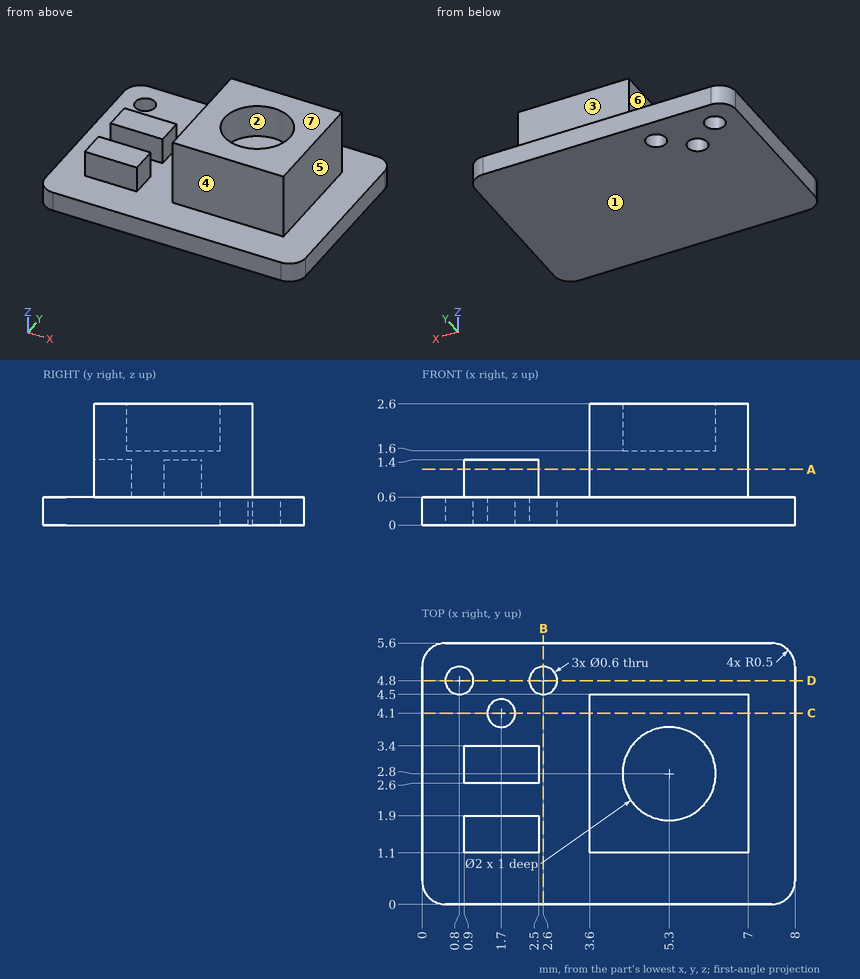
Answer from the drawing. Dimensions are ordinates in mm from the lowest x, y and z of the part. A direction names the side the tool comes from. Give positions to 0.01 mm unless a question says otherwise; leave off trailing zeros. Write each loop counter-clockwise with the first axis right and the second up, starting at its lowest first coordinate (ties: lowest second). Pieces come first, ordered by that corner, then holes.
1) Section A-A (z = 1.2) is taken. Write down the section's boundary in (x, y), and give its area (3 significant figures).
2) Section D-D (y = 4.8) is taken. Write down the section's boundary in (x, z), and give its area (3 significant figures).
3) A tool of negligible diameter and unlimited length cuts with its end or side. For the marked faces 4, 5, 6 and 7, from which of +Z, -Z, +X, -X, +Y, -Y can it reach the whole face along a straight path? Write none if from no direction.
4) Section C-C (y = 4.1) is taken. Write down the section's boundary in (x, z).
5) Section B-B (x = 2.6) is taken. Write down the section's boundary in (y, z).
6) Find the intervals of material crossed by L1, parallel to X at y = 4.8, z = 0.35; L2, parallel to X at y = 4.1, z = 0.45; L3, parallel to Y at x = 5.3, z = 1.9, in increasing order.
7) For a pull along Y with two mould halves and no side action, classify the marked faces 1, 2 and 3 as pulls with the +Y half, pulls with the -Y half, needs draft (parallel to the pull), parting line crosses it, or undercut.
8) Given P1, Ø0.9, axis at x = 2, y = 3, coming from the +Z side; P2, Ø0.6, axis at y = 3, z = 1, coming from the -X side; P3, Ø1, axis at y = 3.5, z = 1, coming from the -X side; P4, Ø0.6, axis at x = 1.5, z = 1, coming from the +Y side, each flat-ended and moving along its own axis, determine where each tip first touches the part or whether it passes through.
Response:
1. outline: (0.9, 1.1) - (2.5, 1.1) - (2.5, 1.9) - (0.9, 1.9) - close; (0.9, 2.6) - (2.5, 2.6) - (2.5, 3.4) - (0.9, 3.4) - close; (3.6, 1.1) - (7, 1.1) - (7, 4.5) - (3.6, 4.5) - close
1. area: 14.1 mm2
2. outline: (0, 0) - (0.5, 0) - (0.5, 0.6) - (0, 0.6) - close; (1.1, 0) - (2.3, 0) - (2.3, 0.6) - (1.1, 0.6) - close; (2.9, 0) - (8, 0) - (8, 0.6) - (2.9, 0.6) - close
2. area: 4.08 mm2
3. face 4: +Z, +X, -X, -Y
3. face 5: +Z, +X, +Y, -Y
3. face 6: +Z, +Y, -Y
3. face 7: +Z, +X, -X, +Y, -Y
4. outline: (0, 0) - (1.4, 0) - (1.4, 0.6) - (0, 0.6) - close; (2, 0) - (8, 0) - (8, 0.6) - (7, 0.6) - (7, 2.6) - (3.6, 2.6) - (3.6, 0.6) - (2, 0.6) - close
5. outline: (0, 0) - (4.5, 0) - (4.5, 0.6) - (0, 0.6) - close; (5.1, 0) - (5.6, 0) - (5.6, 0.6) - (5.1, 0.6) - close
6. L1: x = 0 to 0.5, 1.1 to 2.3, 2.9 to 8
6. L2: x = 0 to 1.4, 2 to 8
6. L3: y = 1.1 to 1.8, 3.8 to 4.5
7. face 1: needs draft
7. face 2: undercut
7. face 3: pulls with the +Y half
8. P1: stops at z = 1.4
8. P2: stops at x = 0.9
8. P3: stops at x = 0
8. P4: stops at y = 3.4
